The listing builds one solid part. Answer for the finished solid, in the listing's coordinates (mm). Face numbers are marked on the shaded views. Give positions to 0.01 mm unless a question says otherwise; leave off trailing zeros. Order: outer loops, then holes, each group sorted by start corner. A loop starts at its lowest first (then second) coordinate and runs counter-clockwise, first axis right, second up.
```python
from build123d import *

# Parameters (mm, degrees)
F0_R     = 43.18
F0_R_2   = 12.7
F1_DEPTH = 19.05
F2_SIZE2 = 0.3402954744
F2_SIZE  = 1.27
F4_D     = 4.3942
F4_DEPTH = 6.35
F4_TIP   = 1.3201508661
F6_D     = 3.4544
F6_DEPTH = 15.24
F6_TIP   = 1.0378064612
F8_D     = 4.4958


with BuildPart() as f1:
    # F0 (on Top) → F1 (new body)
    with BuildSketch(Plane.XY):
        Circle(F0_R)
        Circle(F0_R_2, mode=Mode.SUBTRACT)
    extrude(amount=F1_DEPTH)

    # F2
    f2_edges = [f1.edges().sort_by_distance(p)[0] for p in [
        (-12.7, 0, 19.05),
        (-12.7, 0, 0),
    ]]
    f2_side = f1.faces().sort_by_distance((-12.7, 0, 9.525))[0]
    chamfer(f2_edges, length=F2_SIZE, length2=F2_SIZE2, reference=f2_side)

    # F4
    with Locations(Plane(origin=(0, 0, 0), x_dir=(1, 0, 0), z_dir=(0, 0, -1))):
        with Locations((0, -17.78), (-17.78, 0), (0, 17.78), (17.78, 0)):
            Hole(F4_D / 2, depth=F4_DEPTH)
            with Locations((0, 0, -(F4_DEPTH + F4_TIP / 2))):  # 118° drill point
                Cone(0, F4_D / 2, F4_TIP, mode=Mode.SUBTRACT)

    # F6
    with Locations(Plane.XY.offset(19.05)):
        with Locations((35, 0), (0, -35), (-35, 0), (0, 35)):
            Hole(F6_D / 2, depth=F6_DEPTH)
            with Locations((0, 0, -(F6_DEPTH + F6_TIP / 2))):  # 118° drill point
                Cone(0, F6_D / 2, F6_TIP, mode=Mode.SUBTRACT)

    # F8 (through all)
    with Locations(Plane.XY.offset(19.05)):
        with Locations((24.7487373415, -24.7487373415), (-24.7487373415, -24.7487373415), (-24.7487373415, 24.7487373415), (24.7487373415, 24.7487373415)):
            Hole(F8_D / 2)


solid = f1.part
```
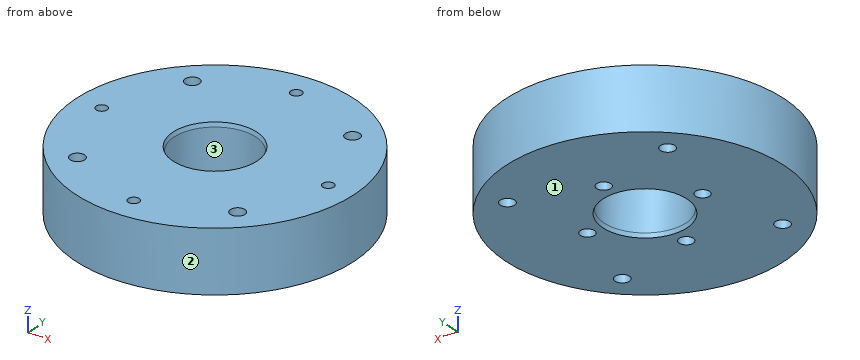
1) Straight lines are drawn through the part: probe 1 along Y at (x, z) = (0, 13.75); probe 2 along X at (y, z) = (24.5, 10); probe 3 along Y at (x, z) = (23.5, 12.5). For each, find the intervals that lie inside material, in ascending order.
Geometry says:
probe 1: y = -43.18 to -36.73, -33.27 to -12.7, 12.7 to 33.27, 36.73 to 43.18
probe 2: x = -35.56 to -26.98, -22.51 to 22.51, 26.98 to 35.56
probe 3: y = -36.23 to -26.62, -22.88 to 22.88, 26.62 to 36.23
2) Find section B-B (z = 16.25). Count the separate pieces of the cut face and the enclosed holes in it, then the cut area to 3 significant figures.
Geometry says:
separate pieces: 1
enclosed holes: 9
area: 5,250 mm2
3) For a pull along X with two mould halves and no side action, classify the marked faces 1, 2 and 3 as +X half, -X half, draft (parallel to the pull), parting line (faces both ways), or undercut.
Geometry says:
face 1: draft
face 2: parting line
face 3: undercut
4) Find section D-D (x = -38). Write down the section's boundary in (y, z), then the cut area to 3 significant figures.
Geometry says:
outline: (-20.51, 0) - (20.51, 0) - (20.51, 19.05) - (-20.51, 19.05) - close
area: 781 mm2
5) Given P1, Ø3.5, axis at x = 24.75, y = 24.75, coming from the -Z side; P2, Ø4, axis at y = 17.5, z = 17, coming from the -X side; P3, Ø10, axis at y = -30.5, z = 5, coming from the -X side; P4, Ø6, axis at x = -22, z = 8.5, coming from the -Y side, each flat-ended and moving along its own axis, determine where each tip first touches the part or whether it passes through.
Geometry says:
P1: passes through
P2: stops at x = -40.3
P3: stops at x = -34.85
P4: stops at y = -38.78
6) Find section A-A (x = -25.5). Write down the section's boundary in (y, z).
Geometry says:
outline: (-34.85, 0) - (-26.87, 0) - (-26.87, 19.05) - (-34.85, 19.05) - close; (-22.63, 0) - (22.63, 0) - (22.63, 19.05) - (-22.63, 19.05) - close; (26.87, 0) - (34.85, 0) - (34.85, 19.05) - (26.87, 19.05) - close
7) Find section C-C (x = 21). Write down the section's boundary in (y, z).
Geometry says:
outline: (-37.73, 0) - (37.73, 0) - (37.73, 19.05) - (-37.73, 19.05) - close
